Could you check a few things on this model? Use its own coordinates, in mm. A direction names the side the tool comes from. Give positions to 0.01 mm unless a question says otherwise; leave off trailing zeros. Order: outer loops, then holes, each group sorted by start corner. A loop starts at its lowest first (then second) coordinate and runs counter-clockwise, first axis right, second up.
(1) If we mould it in two halves opening along Z, with no side actions, what happens to faces 4 (the flat face through (14, -7, 0)), 5 (the cylindrical face through (19.1, -5.7, 0.2)), 6 (the cylindrical face through (11.44, -17.96, -0.54))? For each: released by +Z, released by -Z, zero draft, split by the parting line, or undercut.
(2) On a 3-axis mill with a long thin cutter (end or side, diameter ignored), from which of +Z, -Z, +X, -X, +Y, -Y can I reach the whole of each face in a straight line? I mean faces 1 (the flat face through (-24, -9, 0)), 2 (the flat face through (-21, -7, 0)), 3 (the cylindrical face through (-8.56, -17.96, -0.54)). Say none if no direction works.
(3) Will these pins go through, and if not, where does the flat tip stop? pin 1 (4 mm diameter, centred on x = -6, y = -16.5, fed in from -Z); pin 2 (1 mm diameter, centred on x = 10, z = 5, fed in from -Y); pin 3 (8 mm diameter, centred on x = -13.5, z = -9.5, fed in from +Y).
(4) Imagine slicing it at B-B, the plane y = -16.5. Write out the boundary of the cut face in (x, z).
(5) Imagine slicing it at A-A, the plane x = -11. Write out the boundary of the cut face in (y, z), then the cut area to 3 significant figures.
(6) Imagine slicing it at C-C, the plane z = 0. Write out the boundary of the cut face in (x, y), then the cut area to 3 significant figures.
(7) If I drill on probe 1 along X at (y, z) = (-7.75, -9.5); probe 2 along Y at (x, z) = (9.5, -2); probe 3 along Y at (x, z) = (10, -11), over which ranges is the centre line in solid material (lowest first)?
(8) Imagine slicing it at D-D, the plane y = -4. Write out the boundary of the cut face in (x, z).
from build123d import *

# Parameters (mm, degrees)
SCHIZZO1_W                   = 48
SCHIZZO1_H                   = 31
ESTRUSIONE_ESTRUSIONE1_DEPTH = 15.5
TAGLIO_ESTRUSIONE1_REACH     = 44.157
SCHIZZO2_W                   = 35
SCHIZZO2_H                   = 26
SCHIZZO3_R                   = 21.2
TAGLIO_ESTRUSIONE2_DEPTH     = 53.768361733
SCHIZZO5_W                   = 2.5
SCHIZZO5_H                   = 5
RIPETIZIONE_A_L1_COUNT       = 2
RIPETIZIONE_A_L1_PITCH       = 20


with BuildPart() as part:
    # Schizzo1 → Estrusione-Estrusione1 (new, symmetric)
    with BuildSketch(Plane.XY):
        Rectangle(SCHIZZO1_W, SCHIZZO1_H)
    extrude(amount=ESTRUSIONE_ESTRUSIONE1_DEPTH, both=True)

    # Schizzo2 → Taglio-Estrusione1 (cut, up to next)
    with BuildSketch(Plane.XY.offset(15.5), mode=Mode.PRIVATE) as taglio_estrusione1_sk1:
        with Locations((-3.5, 2.5)):
            Rectangle(SCHIZZO2_W, SCHIZZO2_H)
    taglio_estrusione1_tool1 = extrude(taglio_estrusione1_sk1.sketch, amount=-TAGLIO_ESTRUSIONE1_REACH, mode=Mode.PRIVATE) & part.part
    add(taglio_estrusione1_tool1.solids().sort_by_distance((-3.5, 2.5, 15.5))[0], mode=Mode.SUBTRACT)

    # Schizzo3 → Taglio-Estrusione2 (cut, through all)
    with BuildSketch(Plane(origin=(24, 0, 0), x_dir=(0, 0, -1), z_dir=(1, 0, 0))):
        with Locations((0, 15.5)):
            Circle(SCHIZZO3_R)
    extrude(amount=-TAGLIO_ESTRUSIONE2_DEPTH, mode=Mode.SUBTRACT)

    # Schizzo5 → Rivoluzione2 (revolve)
    with BuildSketch(Plane.XY, mode=Mode.PRIVATE) as rivoluzione2_sk:
        with Locations((10.25, -18)):
            Rectangle(SCHIZZO5_W, SCHIZZO5_H)
    rivoluzione2 = revolve(rivoluzione2_sk.sketch.rotate(Axis((9, -15.5, 0), (0, -1, 0)), 90), axis=Axis((9, -15.5, 0), (0, -1, 0)))

    # Ripetizione a L1: Rivoluzione2 ×2
    with Locations(*[(-i * RIPETIZIONE_A_L1_PITCH, 0, 0) for i in range(1, RIPETIZIONE_A_L1_COUNT)]):
        add(rivoluzione2)


solid = part.part
Answer block:
1. face 4: zero draft
1. face 5: undercut
1. face 6: split by the parting line
2. face 1: +Z, -Z, -X, +Y, -Y
2. face 2: +Z, -Z, +Y
2. face 3: -Y
3. pin 1: stops at z = -15.5
3. pin 2: stops at y = -15.5
3. pin 3: stops at y = -10.5
4. outline: circle Ø5 at (-11, 0); circle Ø5 at (9, 0)
5. outline: (-20.5, -2.5) - (-15.5, -2.5) - (-15.5, -15.5) - (-10.5, -15.5) - (-10.5, 15.5) - (-15.5, 15.5) - (-15.5, 2.5) - (-20.5, 2.5) - close
5. area: 180 mm2
6. outline: (-24, -15.5) - (-13.5, -15.5) - (-13.5, -20.5) - (-8.5, -20.5) - (-8.5, -15.5) - (6.5, -15.5) - (6.5, -20.5) - (11.5, -20.5) - (11.5, -15.5) - (24, -15.5) - (24, -5.7) - (14, -5.7) - (14, -10.5) - (-21, -10.5) - (-21, -5.7) - (-24, -5.7) - close
6. area: 352 mm2
7. probe 1: x = -24 to -21, 14 to 24
7. probe 2: y = -20.5 to -10.5
7. probe 3: y = -15.5 to -10.5
8. outline: (-24, -15.5) - (-21, -15.5) - (-21, -8.32) - (-24, -8.32) - close; (-24, 8.32) - (-21, 8.32) - (-21, 15.5) - (-24, 15.5) - close; (14, -15.5) - (24, -15.5) - (24, -8.32) - (14, -8.32) - close; (14, 8.32) - (24, 8.32) - (24, 15.5) - (14, 15.5) - close
